Design review of the part built by this model. Coordinates are the model's own, in mm. Face numbers are marked on the shaded views. A direction names the side the tool comes from. Round coordinates to 2 decimals unless told otherwise and drop trailing zeros. Write each loop counter-clockwise with the first axis right and the second up, starting at its lowest first coordinate (ties: lowest second). Pieces come first, ordered by that corner, then holes. Notation, with made-up numbers: (33.5, -7.5) - (89.5, -7.5) arc R13 cw to (89.5, 12.5) - close; hole circle Ø1 at (43, 80). An arc over 180 degrees is marked (long way). Use one line per item in the form item = value.
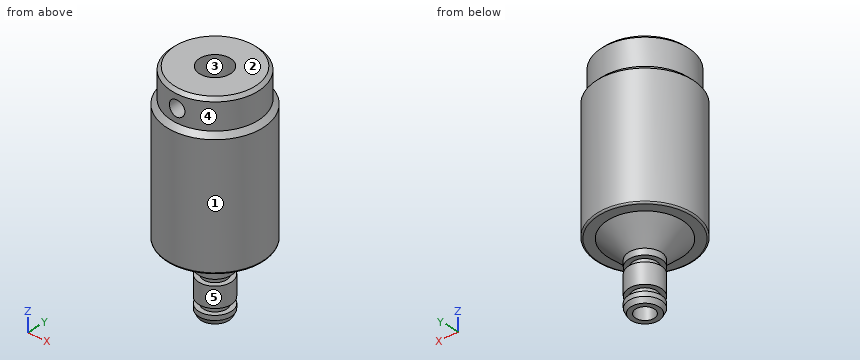
```python
from build123d import *

# Parameters (mm, degrees)
OUTSIDE_BOTTOM_FILLET_R   = 0.25
TOP_CHAMFER_SIZE          = 0.5
M3X0_5_TAPPED_HOLE_REACH  = 39.303
M3X0_5_TAPPED_HOLE_BORE_R = 1.25


with BuildPart() as part:
    # Body Sketch → Body Revolve (revolve)
    with BuildSketch(Plane(origin=(0, 0, 0), x_dir=(1, 0, 0), z_dir=(0, 1, 0)), mode=Mode.PRIVATE) as body_revolve_sk:
        Polygon((2.5, -36), (7, -36), (7, -31.25), (7.75, -30.5), (7.75, -10.9), (6, -10.9), (2.625, -7.75), (2.625, -6.75), (1.875, -6.75), (1.875, -5.75), (2.625, -5.75), (2.625, -2.5), (1.875, -2.5), (1.875, -1.5), (2.625, -1.5), (2.625, -0.75), (2.25, 0), (1.5, 0), (1.5, -30.422649731), (2.5, -31), align=None)
    revolve(body_revolve_sk.sketch.rotate(Axis((0, 0, 0), (0, 0, 1)), 180), axis=Axis((0, 0, 0), (0, 0, 1)))

    # Outside Bottom Fillet
    outside_bottom_fillet_edges = [part.edges().sort_by_distance(p)[0] for p in [
        (7.75, 0, 10.9),
    ]]
    fillet(outside_bottom_fillet_edges, radius=OUTSIDE_BOTTOM_FILLET_R)

    # Top Chamfer
    top_chamfer_edges = [part.edges().sort_by_distance(p)[0] for p in [
        (7, 0, 36),
    ]]
    chamfer(top_chamfer_edges, length=TOP_CHAMFER_SIZE)

    # M3x0.5 Tapped Hole bore (on position points) → M3x0.5 Tapped Hole (cut, up to next)
    with BuildSketch(Plane(origin=(0, -7, 33.375), x_dir=(-1, 0, 0), z_dir=(0, -1, 0)), mode=Mode.PRIVATE) as m3x0_5_tapped_hole_sk1:
        Circle(M3X0_5_TAPPED_HOLE_BORE_R)
    m3x0_5_tapped_hole_tool1 = extrude(m3x0_5_tapped_hole_sk1.sketch, amount=-M3X0_5_TAPPED_HOLE_REACH, mode=Mode.PRIVATE) & part.part
    add(m3x0_5_tapped_hole_tool1.solids().sort_by_distance((0, -7, 33.375))[0], mode=Mode.SUBTRACT)


solid = part.part
```
Q1. To check wall thickness, follow line 1 along Y through (x, z) = (0, 17); line 2 along Z through (x, y) = (2.25, -5.75); line 3 along Z through (x, y) = (0, -4.25) (3 decimals). State the ranges of each line that lie inside material, in increasing order. Write a range as from..to.
Calculated:
line_1 = -7.75..-1.5, 1.5..7.75
line_2 = 10.9..36
line_3 = 9.267..32.125, 34.625..36
Q2. Machinability: for the marked faces 4 and 5, which of the approach directions +Z, -Z, +X, -X, +Y, -Y give a long, thin tool a straight path to every point of the face, cutting with its end or side? Answer none if there is none.
Calculated:
face_4 = +Z
face_5 = -Z
Q3. Draft analysis for pull direction X (two halves, no side actions). For the marked faces 1, 2 and 3, state which applies: released by +X, released by -X, zero draft, split by the parting line, or undercut.
Calculated:
face_1 = split by the parting line
face_2 = zero draft
face_3 = undercut
Q4. We need section C-C on z = 4.5. Write out the cut boundary in (x, y) (3 decimals).
Calculated:
outline = circle Ø5.25 at (0, 0); hole circle Ø3 at (0, 0)
Q5. We need section B-B on z = 19. Write out the cut boundary in (x, y), then the cut area to 3 significant figures.
Calculated:
outline = circle Ø15.5 at (0, 0); hole circle Ø3 at (0, 0)
area = 182 mm2
Q6. For P1, Ø1.6, axis at x = -1, y = 0.5, coming from the +Z side; P2, Ø8, axis at x = -6, z = 27.5, coming from the -Y side; P3, Ø1.8, axis at x = 0, y = 0, coming from the +Z side; P4, Ø6, axis at y = 4, z = 6.5, coming from the -X side, all flat-tipped, find the tip position at first contact; note any pin that passes through.
Calculated:
P1 = 30.66
P2 = -7.49
P3 = through
P4 = -3.21
Q7. We need section A-A on x = 0. State how many separate pieces and enclosed holes the cut face has, then the cut area to 3 significant figures.
Calculated:
separate_pieces = 3
enclosed_holes = 0
area = 316 mm2
